from build123d import *

# Parameters (mm, degrees)
BOSS_EXTRUDE1_DEPTH                             = 38.1
SHELL1_T                                        = -1.6002
BOSS_EXTRUDE2_START                             = 2.2098
BOSS_EXTRUDE2_DEPTH                             = 3.81
FILLET1_R                                       = 2.54
FILLET2_R                                       = 2.54
CUT_EXTRUDE1_REACH                              = 78.617
SKETCH4_W                                       = 19.05
SKETCH4_H                                       = 17.399
CBORE_FOR_2_PAN_HEAD_MACHINE_SCREW1_D           = 2.7051
CBORE_FOR_2_PAN_HEAD_MACHINE_SCREW1_DEPTH       = 1.6002
CBORE_FOR_2_PAN_HEAD_MACHINE_SCREW1_CBORE_D     = 4.7625
CBORE_FOR_2_PAN_HEAD_MACHINE_SCREW1_CBORE_DEPTH = 1.5748
CBORE_FOR_2_PAN_HEAD_MACHINE_SCREW2_D           = 2.7051
CBORE_FOR_2_PAN_HEAD_MACHINE_SCREW2_DEPTH       = 1.6002
CBORE_FOR_2_PAN_HEAD_MACHINE_SCREW2_CBORE_D     = 4.7625
CBORE_FOR_2_PAN_HEAD_MACHINE_SCREW2_CBORE_DEPTH = 1.5748
CBORE_FOR_2_PAN_HEAD_MACHINE_SCREW3_D           = 2.7051
CBORE_FOR_2_PAN_HEAD_MACHINE_SCREW3_DEPTH       = 1.6002
CBORE_FOR_2_PAN_HEAD_MACHINE_SCREW3_CBORE_D     = 4.7625
CBORE_FOR_2_PAN_HEAD_MACHINE_SCREW3_CBORE_DEPTH = 1.5748
CBORE_FOR_2_PAN_HEAD_MACHINE_SCREW4_D           = 2.7051
CBORE_FOR_2_PAN_HEAD_MACHINE_SCREW4_CBORE_D     = 4.7625
CBORE_FOR_2_PAN_HEAD_MACHINE_SCREW4_CBORE_DEPTH = 1.5748
HOLE1_AT_2_COUNT                                = 2
HOLE1_AT_2_PITCH                                = 19
HOLE1_AT_3_COUNT                                = 2
HOLE1_AT_3_PITCH                                = 24.759152348
HOLE1_AT_4_COUNT                                = 2
HOLE1_AT_4_PITCH                                = 15.875
HOLE1_AT_5_COUNT                                = 2
HOLE1_AT_5_PITCH                                = 31.75
HOLE1_AT_6_COUNT                                = 2
HOLE1_AT_6_PITCH                                = 37.000844585
F_0_CLEARANCE_HOLE1_D                           = 1.8542
CUT_EXTRUDE2_REACH                              = 59.194
SKETCH27_R                                      = 6.35


with BuildPart() as part:
    # Sketch1 → Boss-Extrude1 (new body)
    with BuildSketch(Plane.XY):
        with BuildLine():
            Line((-19.03965798, -28.067), (-29.07265798, -18.034))
            Line((-29.07265798, -18.034), (-29.07265798, 18.034))
            Line((-29.07265798, 18.034), (-23.513075374, 23.593582606))
            Line((-23.513075374, 23.593582606), (23.513075374, 23.593582606))
            Line((23.513075374, 23.593582606), (29.07265798, 18.034))
            Line((29.07265798, 18.034), (29.07265798, -6.832479122))
            Line((29.07265798, -6.832479122), (30.1625, -6.832479122))
            Line((30.1625, -6.832479122), (30.1625, -26.9875))
            ThreePointArc((30.1625, -26.9875), (29.23256403, -29.23256403), (26.9875, -30.1625))
            Line((26.9875, -30.1625), (13.90175798, -30.1625))
            Line((13.90175798, -30.1625), (13.90175798, -28.067))
            Line((13.90175798, -28.067), (-19.03965798, -28.067))
        make_face()
    extrude(amount=BOSS_EXTRUDE1_DEPTH)

    # Shell1
    shell1_openings = [part.faces().sort_by_distance(p)[0] for p in [
        (0.895795901, -2.511562828, 0),
    ]]
    offset(amount=SHELL1_T, openings=shell1_openings, kind=Kind.INTERSECTION)

    # Sketch14 → Boss-Extrude2 (add)
    with BuildSketch(Plane(origin=(0, 0, 36.4998), x_dir=(-1, 0, 0), z_dir=(0, 0, -1)).offset(BOSS_EXTRUDE2_START)):
        with BuildLine():
            Line((27.47245798, 17.371175457), (22.850250832, 21.993382606))
            Line((22.850250832, 21.993382606), (-22.850250832, 21.993382606))
            Line((-22.850250832, 21.993382606), (-27.47245798, 17.371175457))
            Line((-27.47245798, 17.371175457), (-27.47245798, -8.432679122))
            Line((-27.47245798, -8.432679122), (-28.5623, -8.432679122))
            Line((-28.5623, -8.432679122), (-28.5623, -26.9875))
            ThreePointArc((-28.5623, -26.9875), (-28.101051759, -28.101051759), (-26.9875, -28.5623))
            Line((-26.9875, -28.5623), (-15.50195798, -28.5623))
            Line((-15.50195798, -28.5623), (-15.50195798, -26.4668))
            Line((-15.50195798, -26.4668), (18.376833438, -26.4668))
            Line((18.376833438, -26.4668), (27.47245798, -17.371175457))
            Line((27.47245798, -17.371175457), (27.47245798, 17.371175457))
        make_face()
    extrude(amount=-BOSS_EXTRUDE2_DEPTH)

    # Fillet1
    # the kernel refuses this fillet: 2.54 mm, written as the material it adds along each edge
    with BuildSketch(Plane(origin=(13.90175798, -28.067, 0), x_dir=(0, -1, 0), z_dir=(0, 0, 1))) as fillet1_piece_1:
        with BuildLine():
            CenterArc((2.54, -2.500803821), FILLET1_R, 100.078658108, 79.921341892)
            Line((0, -2.500803821), (0, 0))
            Line((0, 0), (2.0955, 0))
        make_face()
    extrude(amount=38.1)
    with BuildSketch(Plane(origin=(28.5623, -8.432679122, 34.29), x_dir=(0, -1, 0), z_dir=(0, 0, -1))) as fillet1_piece_2:
        with BuildLine():
            CenterArc((2.08533974, 2.54), FILLET1_R, 214.814987039, 55.185012961)
            Line((0, 1.08984202), (0, 0))
            Line((0, 0), (2.08533974, 0))
        make_face()
    extrude(amount=34.29)
    with BuildSketch(Plane(origin=(29.07265798, -6.832479122, 0), x_dir=(0, 1, 0), z_dir=(0, 0, 1))) as fillet1_piece_3:
        with BuildLine():
            CenterArc((2.08533974, -2.54), FILLET1_R, 90, 55.185012961)
            Line((0, -1.08984202), (0, 0))
            Line((0, 0), (2.08533974, 0))
        make_face()
    extrude(amount=38.1)
    # the kernel refuses this fillet: 2.54 mm, written as the material it takes off along each edge
    with BuildSketch(Plane(origin=(15.50195798, -26.4668, -6.252009552), x_dir=(-1, 0, 0), z_dir=(0, 0, 1))) as fillet1_2_piece_1:
        with BuildLine():
            CenterArc((2.500803821, 2.54), FILLET1_R, 190.078658108, 79.921341892)
            Line((0, 2.0955), (0, 0))
            Line((0, 0), (2.500803821, 0))
        make_face()
    extrude(amount=40.542009552, mode=Mode.SUBTRACT)
    with BuildSketch(Plane(origin=(-29.07265798, -18.034, -2.630256121), x_dir=(0.7071067811865475, -0.7071067811865475, 0), z_dir=(0, 0, 1)), Plane(origin=(-19.03965798, -28.067, -2.630256121), x_dir=(1, 0, 0), z_dir=(0, 0, 1)), Plane(origin=(29.07265798, 18.034, -2.630256121), x_dir=(-0.7071067811865476, 0.7071067811865476, 0), z_dir=(0, 0, 1)), Plane(origin=(23.513075374, 23.593582606, -2.630256121), x_dir=(-1, 0, 0), z_dir=(0, 0, 1)), Plane(origin=(-23.513075374, 23.593582606, -2.630256121), x_dir=(-0.7071067811865476, -0.7071067811865476, 0), z_dir=(0, 0, 1)), Plane(origin=(-29.07265798, 18.034, -2.630256121), x_dir=(0, -1, 0), z_dir=(0, 0, 1))) as fillet1_2_piece_2:
        with BuildLine():
            CenterArc((FILLET1_R * 0.414213562373, FILLET1_R), FILLET1_R, 225, 45)
            Line((-FILLET1_R * 0.292893218813, FILLET1_R * 0.292893218813), (0, 0))
            Line((0, 0), (FILLET1_R * 0.414213562373, 0))
        make_face()
    extrude(amount=43.360512242, mode=Mode.SUBTRACT)

    # Fillet2
    fillet2_edges = [part.edges().sort_by_distance(p)[0] for p in [
        (30.1625, -6.832479122, 19.05),
        (13.90175798, -30.1625, 19.05),
        (27.47245798, -8.432679122, 17.145),
        (15.50195798, -28.5623, 17.145),
    ]]
    fillet(fillet2_edges, radius=FILLET2_R)

    # Sketch4 → Cut-Extrude1 (cut, up to next)
    with BuildSketch(Plane(origin=(30.1625, 0, 0), x_dir=(0, 0, -1), z_dir=(1, 0, 0)), mode=Mode.PRIVATE) as cut_extrude1_sk1:
        with Locations((-9.525, -19.8628)):
            Rectangle(SKETCH4_W, SKETCH4_H)
    cut_extrude1_tool1 = extrude(cut_extrude1_sk1.sketch, amount=-CUT_EXTRUDE1_REACH, mode=Mode.PRIVATE) & part.part
    add(cut_extrude1_tool1.solids().sort_by_distance((30.1625, -19.8628, 9.525))[0], mode=Mode.SUBTRACT)

    # CBORE for #2 Pan Head Machine Screw1
    with Locations(Plane.ZY.offset(29.07265798)):
        with Locations((3.6565, 0)):
            CounterBoreHole(CBORE_FOR_2_PAN_HEAD_MACHINE_SCREW1_D / 2, CBORE_FOR_2_PAN_HEAD_MACHINE_SCREW1_CBORE_D / 2, CBORE_FOR_2_PAN_HEAD_MACHINE_SCREW1_CBORE_DEPTH, depth=CBORE_FOR_2_PAN_HEAD_MACHINE_SCREW1_DEPTH)

    # CBORE for #2 Pan Head Machine Screw2
    with Locations(Plane(origin=(0, 23.593582606, 0), x_dir=(1, 0, 0), z_dir=(0, 1, 0))):
        with Locations((0, -3.6565)):
            CounterBoreHole(CBORE_FOR_2_PAN_HEAD_MACHINE_SCREW2_D / 2, CBORE_FOR_2_PAN_HEAD_MACHINE_SCREW2_CBORE_D / 2, CBORE_FOR_2_PAN_HEAD_MACHINE_SCREW2_CBORE_DEPTH, depth=CBORE_FOR_2_PAN_HEAD_MACHINE_SCREW2_DEPTH)

    # CBORE for #2 Pan Head Machine Screw3
    with Locations(Plane(origin=(29.07265798, 0, 0), x_dir=(0, 0, -1), z_dir=(1, 0, 0))):
        with Locations((-3.6565, 10.957528192)):
            CounterBoreHole(CBORE_FOR_2_PAN_HEAD_MACHINE_SCREW3_D / 2, CBORE_FOR_2_PAN_HEAD_MACHINE_SCREW3_CBORE_D / 2, CBORE_FOR_2_PAN_HEAD_MACHINE_SCREW3_CBORE_DEPTH, depth=CBORE_FOR_2_PAN_HEAD_MACHINE_SCREW3_DEPTH)

    # CBORE for #2 Pan Head Machine Screw4 (through all)
    with Locations(Plane(origin=(0, -28.067, 0), x_dir=(-1, 0, 0), z_dir=(0, -1, 0))):
        with Locations((0, -3.6565)):
            CounterBoreHole(CBORE_FOR_2_PAN_HEAD_MACHINE_SCREW4_D / 2, CBORE_FOR_2_PAN_HEAD_MACHINE_SCREW4_CBORE_D / 2, CBORE_FOR_2_PAN_HEAD_MACHINE_SCREW4_CBORE_DEPTH)

    # Sketch24 → Hole1 (revolve, cut)
    with BuildSketch(Plane(origin=(9.5, 13.49375, 34.29), x_dir=(0, 1, 0), z_dir=(1, 0, 0))):
        Polygon((0, 0), (0, 2.921), (1.4986, 2.921), (1.6383, 0), align=None)
    hole1 = revolve(axis=Axis((9.5, 13.49375, 144.29), (0, 0, -1)), mode=Mode.SUBTRACT)

    # Hole1 at 2: Hole1 ×2
    with Locations(*[(-i * HOLE1_AT_2_PITCH, 0, 0) for i in range(1, HOLE1_AT_2_COUNT)]):
        add(hole1, mode=Mode.SUBTRACT)

    # Hole1 at 3: Hole1 ×2
    with Locations(*[Vector(-0.7673929920061523, -0.6411770393735614, 0) * (i * HOLE1_AT_3_PITCH) for i in range(1, HOLE1_AT_3_COUNT)]):
        add(hole1, mode=Mode.SUBTRACT)

    # Hole1 at 4: Hole1 ×2
    with Locations(*[(0, -i * HOLE1_AT_4_PITCH, 0) for i in range(1, HOLE1_AT_4_COUNT)]):
        add(hole1, mode=Mode.SUBTRACT)

    # Hole1 at 5: Hole1 ×2
    with Locations(*[(0, -i * HOLE1_AT_5_PITCH, 0) for i in range(1, HOLE1_AT_5_COUNT)]):
        add(hole1, mode=Mode.SUBTRACT)

    # Hole1 at 6: Hole1 ×2
    with Locations(*[Vector(-0.5135017920030289, -0.8580885208471666, 0) * (i * HOLE1_AT_6_PITCH) for i in range(1, HOLE1_AT_6_COUNT)]):
        add(hole1, mode=Mode.SUBTRACT)

    # #0 Clearance Hole1 (through all)
    with Locations(Plane(origin=(0, 0, 34.29), x_dir=(-1, 0, 0), z_dir=(0, 0, -1))):
        with Locations((-9.5, 13.49375), (9.5, 13.49375), (-9.5, -2.38125), (9.5, -2.38125), (-9.5, -18.25625), (9.5, -18.25625)):
            Hole(F_0_CLEARANCE_HOLE1_D / 2)

    # Sketch27 → Cut-Extrude2 (cut, up to next)
    with BuildSketch(Plane.XY.offset(38.1), mode=Mode.PRIVATE) as cut_extrude2_sk1:
        with Locations((0, 13.49375)):
            Circle(SKETCH27_R)
    cut_extrude2_tool1 = extrude(cut_extrude2_sk1.sketch, amount=-CUT_EXTRUDE2_REACH, mode=Mode.PRIVATE) & part.part
    # Sketch27 → Cut-Extrude2 (cut, up to next)
    with BuildSketch(Plane.XY.offset(38.1), mode=Mode.PRIVATE) as cut_extrude2_sk2:
        with Locations((0, -2.38125)):
            Circle(SKETCH27_R)
    cut_extrude2_tool2 = extrude(cut_extrude2_sk2.sketch, amount=-CUT_EXTRUDE2_REACH, mode=Mode.PRIVATE) & part.part
    # Sketch27 → Cut-Extrude2 (cut, up to next)
    with BuildSketch(Plane.XY.offset(38.1), mode=Mode.PRIVATE) as cut_extrude2_sk3:
        with Locations((0, -18.28125)):
            Circle(SKETCH27_R)
    cut_extrude2_tool3 = extrude(cut_extrude2_sk3.sketch, amount=-CUT_EXTRUDE2_REACH, mode=Mode.PRIVATE) & part.part
    add(cut_extrude2_tool1.solids().sort_by_distance((0, 13.49375, 38.1))[0], mode=Mode.SUBTRACT)
    add(cut_extrude2_tool2.solids().sort_by_distance((0, -2.38125, 38.1))[0], mode=Mode.SUBTRACT)
    add(cut_extrude2_tool3.solids().sort_by_distance((0, -18.28125, 38.1))[0], mode=Mode.SUBTRACT)


solid = part.part
Part model, mm, in its own coordinate system. A direction names the side the tool comes from. Coordinates: 2 decimals unless noted, no trailing zeros. Order: outer loops, then holes, each group sorted by start corner. A loop starts at its lowest first (then second) coordinate and runs counter-clockwise, first axis right, second up. Notation, with made-up numbers: M 53.5,-16 L 78.5,-16 A22 cw 78.5,13 Z; hole C -12.75,-40 d10. An arc over 180 degrees is marked long. One line per question, with ' | ' between items.
Q1. Pin check, flat tips, straight feed: P1, Ø1.8, axis at x = 29.5, z = 8, coming from the -Y side; P2, Ø3, axis at y = 0, z = 3.66, coming from the +X side; P3, Ø12, axis at x = 4.5, y = 16, coming from the +Z side; P4, Ø1.5, axis at x = 10, y = -18, coming from the -Z side. Stop position of each tip, or through.
A:
P1: stops at y = -29.72 | P2: stops at x = 29.07 | P3: stops at z = 38.1 | P4: stops at z = 37.21
Q2. Slice it at C-C (y = 5). Give the cut face in (x, z), and give its area (3 significant figures).
A:
outline: M -29.07,0 L -27.47,0 L -27.47,34.29 L 27.47,34.29 L 27.47,0 L 29.07,0 L 29.07,38.1 L -29.07,38.1 Z | area: 331 mm^2
Q3. Slice it at D-D (y = -5.5). Give the cut face in (x, z), and give its area (3 significant figures).
A:
outline: M -29.07,0 L -27.47,0 L -27.47,34.29 L -5.53,34.29 L -5.53,38.1 L -29.07,38.1 Z; M 5.53,34.29 L 27.47,34.29 L 27.47,0 L 29.19,0 L 29.19,38.1 L 5.53,38.1 Z | area: 293 mm^2
Q4. Slice it at A-A (x = -9.5). Count the separate pieces of the cut face and the enclosed holes in it, and give its area (3 significant figures).
A:
separate pieces: 4 | enclosed holes: 0 | area: 274 mm^2
Q5. 3-axis set-ups, long thin cutter, end or side, ignore diameter. For faces 1 (the face through (29, -11.163, 10)), 2 (the face through (28.3, 13.32, 3.97)), 3 (the face through (23.446, 23.395, 18.783)), 4 (the face through (-27.472, 0, 17)): which of +Z, -Z, +X, -X, +Y, -Y reach the whole face in a straight line?
A:
face 1: -Z, +X | face 2: +X | face 3: +Z, -Z, +X, +Y | face 4: -Z
Q6. Drill centre lines: line 1 (Y direction, x = 0, z = 35); line 2 (Y direction, x = 17, z = 5.5); line 3 (Y direction, x = -8, z = 16.5). Where is each one in solid material? Low to high.
A:
line 1: y = -28.07 to -24.63, -11.93 to -8.73, 3.97 to 7.14, 19.84 to 23.59 | line 2: y = -30.16 to -28.56, 21.99 to 23.59 | line 3: y = -28.07 to -26.47, 21.99 to 23.59
Q7. Two-plate mould, pull along Z, no slides. Class faces 5 (the face through (-9.431, 11.926, 35.73)), 6 (the face through (0.52, -27.29, 5.98)), 7 (the face through (-28.874, 17.967, 18.783)): +Z half, -Z half, draft (parallel to the pull), parting line (faces both ways), or undercut.
A:
face 5: -Z half | face 6: undercut | face 7: draft
